Input: part model. Units: mm. Frame: model coordinates. Face numbers are marked on the shaded views. Give positions to 0.01 mm unless a question says otherwise; leave off trailing zeros. Loops run counter-clockwise (first coordinate to the right, second up) from the corner with the lowest first, then second, coordinate; pieces in that order, holes last. Notation, with made-up numbers: (-37.75, 2.5) - (0.25, 2.5) arc R5 ccw to (0.25, 8.5) - close; hole circle Ø9 at (-13.5, 67). An arc over 180 degrees is marked (long way). Answer as a JSON object with one key per item and string values.
from build123d import *

# Parameters (mm, degrees)
BOSS_EXTRUDE1_DEPTH = 25


with BuildPart() as part:
    # Sketch1 → Boss-Extrude1 (new body)
    with BuildSketch(Plane(origin=(0, 0, 0), x_dir=(1, 0, 0), z_dir=(0, 1, 0))):
        Polygon((1.732050808, 3), (-1.732050808, 3), (-3.464101615, 0), (-1.732050808, -3), (1.732050808, -3), (3.464101615, 0), align=None)
    extrude(amount=BOSS_EXTRUDE1_DEPTH)

    # Sketch2 → M4 Tapped Hole1 (revolve, cut)
    with BuildSketch(Plane(origin=(0, 25, 0), x_dir=(0, 0, 1), z_dir=(1, 0, 0))):
        Polygon((0, 0), (0, 25), (2.025, 25), (1.65, 24.625), (1.65, 0.375), (2.025, 0), align=None)
    revolve(axis=Axis((0, 31.35, 0), (0, -1, 0)), mode=Mode.SUBTRACT)

    # Sketch4 → Cut-Revolve1 (revolve, cut)
    with BuildSketch(Plane.XY):
        Polygon((2.85, 0), (3.464101615, 0.614101615), (3.464101615, 0), align=None)
        Polygon((3.464101615, 25), (2.85, 25), (3.464101615, 24.385898385), align=None)
    revolve(axis=Axis((0, 25, 0), (0, -1, 0)), mode=Mode.SUBTRACT)


solid = part.part
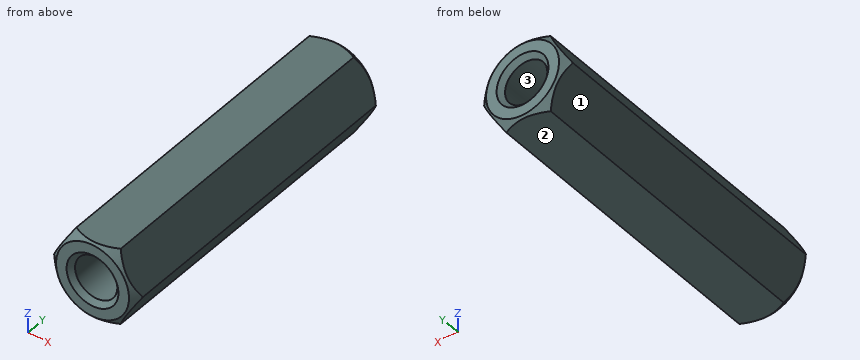
Item 1: Cut plane B-B (y = 3). Return loops of the section in (x, z).
Geometry check:
{"outline": "(-3.46, 0) - (-1.73, -3) - (1.73, -3) - (3.46, 0) - (1.73, 3) - (-1.73, 3) - close; hole circle Ø3.3 at (0, 0)"}
Item 2: Material intervals for line 1 (Z direction, x = 0, y = 6.5); line 2 (Z direction, x = 0.75, y = 11.5); line 3 (X direction, y = 1, z = -0.65), sorted ascending. Write a range as [from, to].
Geometry check:
{"line 1": "z = [-3, -1.65], [1.65, 3]", "line 2": "z = [-3, -1.47], [1.47, 3]", "line 3": "x = [-3.09, -1.52], [1.52, 3.09]"}
Item 3: Cut plane A-A (x = 0). Return loops of the section in (y, z) (3 decimals).
Geometry check:
{"outline": "(0, -2.85) - (0.15, -3) - (24.85, -3) - (25, -2.85) - (25, -2.025) - (24.625, -1.65) - (0.375, -1.65) - (0, -2.025) - close; (0, 2.025) - (0.375, 1.65) - (24.625, 1.65) - (25, 2.025) - (25, 2.85) - (24.85, 3) - (0.15, 3) - (0, 2.85) - close"}
Item 4: Mould query, pull axis X, two halves, no side actions, for the marked faces 1, 2 and 3. Classes: released by +X, released by -X, zero draft, split by the parting line, or undercut.
Geometry check:
{"face 1": "released by -X", "face 2": "zero draft", "face 3": "undercut"}
